Input: part model. Units: mm. Frame: model coordinates. Face numbers are marked on the shaded views. A direction names the side the tool comes from. Round coordinates to 2 decimals unless told otherwise and drop trailing zeros. Write each loop counter-clockwise with the first axis right and the second up, starting at its lowest first coordinate (ties: lowest second). Pieces come first, ordered by that corner, then holes. Notation, with made-up numbers: (86, 42) -> (96, 42) arc R28 ccw to (96, 72) -> close; hole circle Ø8 at (-37.5, -0.5). An arc over 180 degrees is marked (long way). Write item = value, one per line.
Autodesk Inventor part; units mm, degrees
ref_plane "YZ Plane" through (0, 0, 0) normal (1, 0, 0) x (0, 1, 0)
ref_plane "XZ Plane" through (0, 0, 0) normal (0, 1, 0) x (-1, 0, 0)
ref_plane "XY Plane" through (0, 0, 0) normal (0, 0, 1) x (1, 0, 0)
sketch "Sketch1" plane through (0, 0, 0) normal (1, 0, 0) x (0, 1, 0)
  line L0 (-21, 41) -> (21, 41) construction
  line L1 (-5, 36) -> (-5, 10.198)
  line L2 (5, 36) -> (5, 10.198)
  arc A0 (-6.6, 6.1188) -> (6.6, 6.1188) centre (0, 0) ccw
  arc A1 (-6.6, 6.1188) -> (-5, 10.198) centre (-11, 10.198) ccw
  arc A2 (5, 10.198) -> (6.6, 6.1188) centre (11, 10.198) ccw
  arc A3 (-5, 45.7275) -> (5.2222, 45.7026) centre (0, 0) ccw construction
  circle A4 centre (0, 0) radius 1.5
  line L3 (-3, 38) -> (3, 38)
  arc A5 (-3, 38) -> (-5, 36) centre (-3, 36) ccw
  arc A6 (5, 36) -> (3, 38) centre (3, 36) ccw
  point P0 (-5, 38)
  point P1 (5, 38)
  point P2 (-5, 7.4833)
  point P3 (5, 7.4833)
  dimension "d25" = 10
  dimension "d69" = 6
  dimension "d101" = 3
  dimension "d108" = 9
  dimension "d109" = 38
  dimension "d110" = 5
  dimension "d111" = 2
extrude "Extrusion6" add sketch "Sketch1" along normal blind 3
properties part number "Camera Mount_A073113"
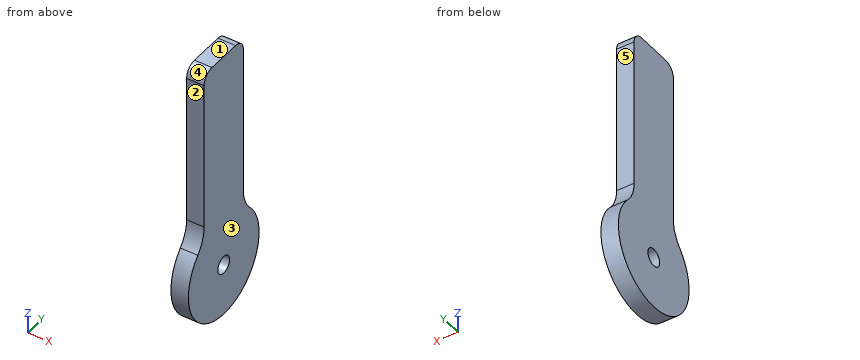
1) Access query for the marked faces 1 and 2. Directions: +Z, -Z, +X, -X, +Y, -Y. A direction counts if a zero-diameter tool reaches every point of the face in a straight line with its end or side. Return the directions, or none.
Solutions:
face_1 = +Z, +X, -X, +Y, -Y
face_2 = +Z, +X, -X, -Y
2) Cut plane A-A (y = 0). Return the cut outline in (x, z), and give its area (3 significant figures).
Solutions:
outline = (0, -9) -> (3, -9) -> (3, -1.5) -> (0, -1.5) -> close; (0, 1.5) -> (3, 1.5) -> (3, 38) -> (0, 38) -> close
area = 132 mm^2
3) Cut plane B-B (z = 0). Return the cut outline in (x, y).
Solutions:
outline = (0, -9) -> (3, -9) -> (3, -1.5) -> (0, -1.5) -> close; (0, 1.5) -> (3, 1.5) -> (3, 9) -> (0, 9) -> close
4) Cut plane C-C (x = 0.7). Return the cut outline in (y, z), and give its area (3 significant figures).
Solutions:
outline = (-6.6, 6.12) arc R9 ccw (long way) to (6.6, 6.12) arc R6 cw to (5, 10.2) -> (5, 36) arc R2 ccw to (3, 38) -> (-3, 38) arc R2 ccw to (-5, 36) -> (-5, 10.2) arc R6 cw to start; hole circle Ø3 at (0, 0)
area = 542 mm^2
5) Draft query along Y for the marked faces 3, 4 and 5. Return one class per face: +Y half, -Y half, draft (parallel to the pull), parting line (faces both ways), or undercut.
Solutions:
face_3 = draft
face_4 = -Y half
face_5 = +Y half
6) Line query: L1, parallel to Z at x = 1.8, y = 0; L2, parallel to Y at x = 1.85, z = 23.5; L3, parallel to Z at x = 1.8, y = 1. Output: solid intervals per line, ascending. Write a range as from..to.
Solutions:
L1 = -9..-1.5, 1.5..38
L2 = -5..5
L3 = -8.94..-1.12, 1.12..38
